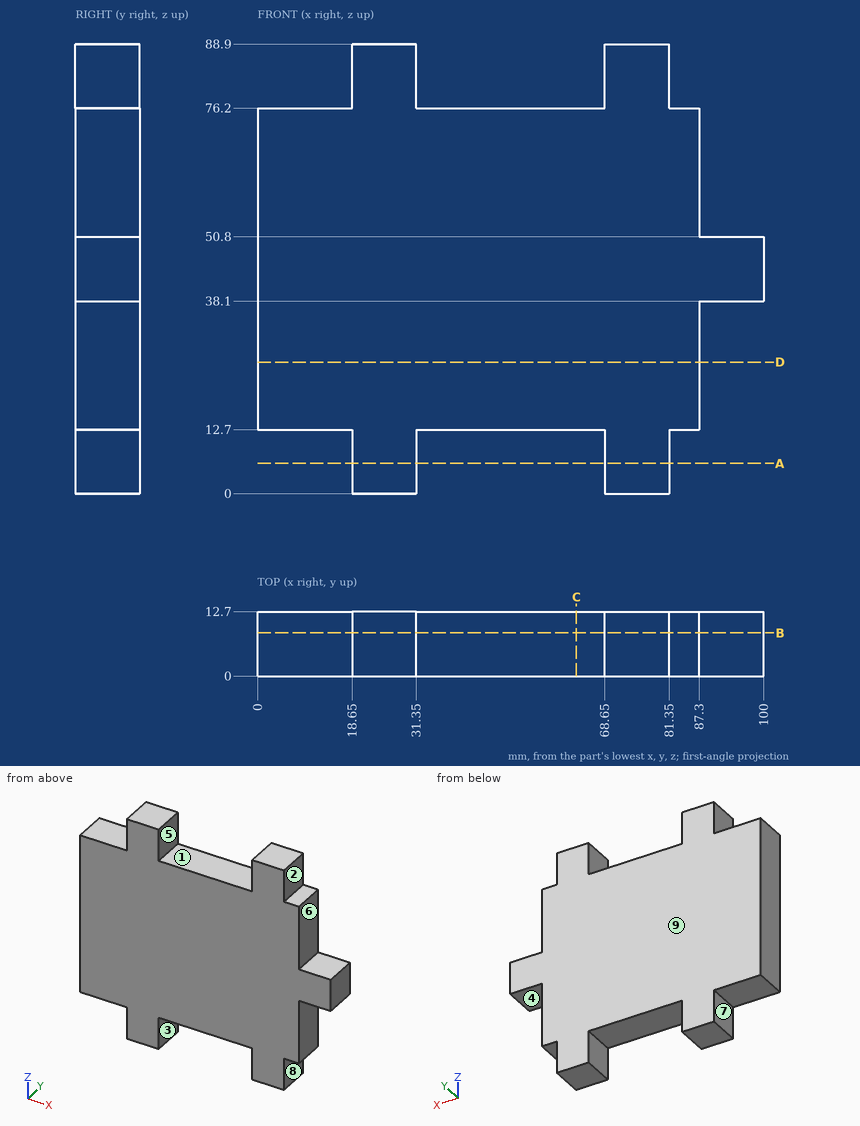
Design review of the part shown in the three views and the two pictorial views. Dimensions are in mm from the part's minimum x, y and z. A direction names the side the tool comes from. Give positions to 0.01 mm unless a question says otherwise; leave off trailing zeros. Order: outer loops, then holes, each group sorted by start corner. A loop starts at its lowest first (then second) coordinate and runs counter-clockwise, first axis right, second up. Notation, with made-up numbers: M -24.5,-18 L -12.5,-18 A16 cw -12.5,-1 Z; hole C 38.25,-25.75 d4. An arc over 180 degrees is marked long. Answer in a Markdown table with one row per item. Add a question column.
(1) Wall thickness on probe 1 along X at (y, z) = (1, 34); probe 2 along Z at (x, y) = (89, 2.75); probe 3 along Z at (x, y) = (41.5, 4.5): over which ranges is each line inside the solid? List them lowest first. Write a range as [from, to].
(2) For pin 1 (4 mm diameter, centred on x = 96.5, y = 8.5, fed in from +Z); pin 2 (5 mm diameter, centred on y = 4, z = 10.5, fed in from +X); pin 3 (5 mm diameter, centred on x = 44.5, y = 5.5, fed in from -Z), all flat-tipped, find the tip position at first contact; note any pin that passes through.
(3) Mouldability with a two-part tool opening along X and no side actions: class the marked faces 1, 2, 3 and 4 as +X half, -X half, draft (parallel to the pull), parting line (faces both ways), or undercut.
(4) Consider section A-A on z = 6. State the section outline as (x, y) points, and give its area (3 significant figures).
(5) For the marked faces 5, 6, 7, 8 and 9, list the 3-axis set-ups (+Z, -Z, +X, -X, +Y, -Y) from which the entire face can be reached by the end or side of a thin tool; tool diameter is ignored.
(6) Consider section C-C on x = 63. State the section outline as (y, z) points.
(7) Consider section B-B on y = 8.5. State the section outline as (x, z) points.
(8) Consider section D-D on z = 26. State the section outline as (x, y) points, and give its area (3 significant figures).
Evaluation:
| question | item | result |
|---|---|---|
| 1 | probe 1 | x = [0, 87.3] |
| 1 | probe 2 | z = [38.1, 50.8] |
| 1 | probe 3 | z = [12.7, 76.2] |
| 2 | pin 1 | stops at z = 50.8 |
| 2 | pin 2 | stops at x = 87.3 |
| 2 | pin 3 | stops at z = 12.7 |
| 3 | face 1 | undercut |
| 3 | face 2 | +X half |
| 3 | face 3 | undercut |
| 3 | face 4 | draft |
| 4 | outline | M 18.65,0 L 31.35,0 L 31.35,12.7 L 18.65,12.7 Z; M 68.65,0 L 81.35,0 L 81.35,12.7 L 68.65,12.7 Z |
| 4 | area | 323 mm^2 |
| 5 | face 5 | +Z, +Y, -Y |
| 5 | face 6 | +Z, +X, +Y, -Y |
| 5 | face 7 | -Z, -X, +Y, -Y |
| 5 | face 8 | -Z, +X, +Y, -Y |
| 5 | face 9 | +Z, -Z, +X, -X, +Y |
| 6 | outline | M 0,12.7 L 12.7,12.7 L 12.7,76.2 L 0,76.2 Z |
| 7 | outline | M 0,12.7 L 18.65,12.7 L 18.65,0 L 31.35,0 L 31.35,12.7 L 68.65,12.7 L 68.65,0 L 81.35,0 L 81.35,12.7 L 87.3,12.7 L 87.3,38.1 L 100,38.1 L 100,50.8 L 87.3,50.8 L 87.3,76.2 L 81.35,76.2 L 81.35,88.9 L 68.65,88.9 L 68.65,76.2 L 31.35,76.2 L 31.35,88.9 L 18.65,88.9 L 18.65,76.2 L 0,76.2 Z |
| 8 | outline | M 0,0 L 87.3,0 L 87.3,12.7 L 0,12.7 Z |
| 8 | area | 1,110 mm^2 |
